Part model, mm, in its own coordinate system. Coordinates: 2 decimals unless noted, no trailing zeros. Order: outer loops, then holes, each group sorted by start corner. A loop starts at its lowest first (then second) coordinate and runs counter-clockwise, first axis right, second up.
from build123d import *

# Parameters (mm, degrees)
SKETCH_1_R               = 31.5
SKETCH_1_R_2             = 22.5
EXTRUDE_1_DEPTH          = 4
SKETCH_2_R               = 2.025
CUT_EXTRUDE_1_DEPTH      = 1
CUT_EXTRUDE_1_DEPTH_BACK = 5
SKETCH_3_R               = 22.5
EXTRUDE_2_DEPTH          = 4
SKETCH_4_R               = 1.525
CUT_EXTRUDE_2_DEPTH      = 4
SKETCH_5_R               = 10
CUT_EXTRUDE_3_DEPTH      = 4


with BuildPart() as part:
    # 草图1 → 凸台-拉伸1 (new body)
    with BuildSketch(Plane(origin=(0, 0, 0), x_dir=(1, 0, 0), z_dir=(0, 1, 0))):
        Circle(SKETCH_1_R)
        Circle(SKETCH_1_R_2, mode=Mode.SUBTRACT)
    extrude(amount=EXTRUDE_1_DEPTH)

    # 草图2 → 切除-拉伸1 (cut, two sides)
    with BuildSketch(Plane(origin=(0, 4, 0), x_dir=(1, 0, 0), z_dir=(0, 1, 0))) as cut_extrude_1_sk:
        with Locations((0, 26.25)):
            Circle(SKETCH_2_R)
        with Locations((18.561553006, 18.561553006)):
            Circle(SKETCH_2_R)
        with Locations((26.25, 0)):
            Circle(SKETCH_2_R)
        with Locations((18.561553006, -18.561553006)):
            Circle(SKETCH_2_R)
        with Locations((0, -26.25)):
            Circle(SKETCH_2_R)
        with Locations((-18.561553006, -18.561553006)):
            Circle(SKETCH_2_R)
        with Locations((-26.25, 0)):
            Circle(SKETCH_2_R)
        with Locations((-18.561553006, 18.561553006)):
            Circle(SKETCH_2_R)
    extrude(amount=CUT_EXTRUDE_1_DEPTH, mode=Mode.SUBTRACT)
    extrude(cut_extrude_1_sk.sketch, amount=-CUT_EXTRUDE_1_DEPTH_BACK, mode=Mode.SUBTRACT)

    # 草图3 → 凸台-拉伸2 (add)
    with BuildSketch(Plane(origin=(0, 4, 0), x_dir=(1, 0, 0), z_dir=(0, 1, 0))):
        Circle(SKETCH_3_R)
    extrude(amount=-EXTRUDE_2_DEPTH)

    # 草图4 → 切除-拉伸2 (cut)
    with BuildSketch(Plane.XZ):
        with Locations((0, 13.5)):
            Circle(SKETCH_4_R)
        with Locations((11.691342951, 6.75)):
            Circle(SKETCH_4_R)
        with Locations((11.691342951, -6.75)):
            Circle(SKETCH_4_R)
        with Locations((0, -13.5)):
            Circle(SKETCH_4_R)
        with Locations((-11.691342951, -6.75)):
            Circle(SKETCH_4_R)
        with Locations((-11.691342951, 6.75)):
            Circle(SKETCH_4_R)
    extrude(amount=-CUT_EXTRUDE_2_DEPTH, mode=Mode.SUBTRACT)

    # 草图5 → 切除-拉伸3 (cut)
    with BuildSketch(Plane.XZ):
        Circle(SKETCH_5_R)
    extrude(amount=-CUT_EXTRUDE_3_DEPTH, mode=Mode.SUBTRACT)


solid = part.part
Q1. Pin check, flat tips, straight feed: pin 1 Ø2 at (y, z) = (1.5, -14) entering from -X; pin 2 Ø1 at (x, y) = (15.5, 1) entering from -Z. Stop position of each tip, or through.
Results list:
pin 1: stops at x = -28.69
pin 2: stops at z = -27.7
Q2. Cut at A-A on z = 0. Write the cut outline in (x, y) (3 decimals).
Results list:
outline: (-31.5, 0) - (-28.275, 0) - (-28.275, 4) - (-31.5, 4) - close; (-24.225, 0) - (-10, 0) - (-10, 4) - (-24.225, 4) - close; (10, 0) - (24.225, 0) - (24.225, 4) - (10, 4) - close; (28.275, 0) - (31.5, 0) - (31.5, 4) - (28.275, 4) - close
Q3. Cut at B-B on z = -26.25. Write the cut outline in (x, y) (3 decimals), and give its area (3 significant figures).
Results list:
outline: (-17.412, 0) - (-2.025, 0) - (-2.025, 4) - (-17.412, 4) - close; (2.025, 0) - (17.412, 0) - (17.412, 4) - (2.025, 4) - close
area: 123 mm2
Q4. Mould opens along X. For faces 1 (the face through (-0.33, 1.97, 12.01)), 2 (the face through (-4.101, 1.972, -31.232)), 3 (the face through (-20.17, 2.03, -17.33)), 4 (the face through (-7.4, 4, -7.4)) say: pulls with the +X half, pulls with the -X half, needs draft (parallel to the pull), parting line crosses it, or undercut.
Results list:
face 1: undercut
face 2: parting line crosses it
face 3: undercut
face 4: needs draft
Q5. Cut at C-C on x = -9. Write the cut outline in (y, z).
Results list:
outline: (0, -30.19) - (4, -30.19) - (4, -4.36) - (0, -4.36) - close; (0, 4.36) - (4, 4.36) - (4, 30.19) - (0, 30.19) - close
Q6. Wall check: line 1 along Z through (x, y) = (0, 1) (3 decimals); line 2 along Z through (x, y) = (-12.5, 0.95); line 3 along X through (y, z) = (1.05, 19). Give the ranges that are in metal, low to high.
Results list:
line 1: z = -31.5 to -28.275, -24.225 to -15.025, -11.975 to -10, 10 to 11.975, 15.025 to 24.225, 28.275 to 31.5
line 2: z = -28.91 to -8.04, -5.46 to 5.46, 8.04 to 28.91
line 3: x = -25.12 to -20.54, -16.58 to 16.58, 20.54 to 25.12
Q7. Cut at D-D on y = 3.25. Count the separate pieces of the cut face and the enclosed holes in it, and give its area (3 significant figures).
Results list:
separate pieces: 1
enclosed holes: 15
area: 2,660 mm2
